The model under review builds one solid part; all positions refer to its coordinate system, in mm. Round coordinates to 2 decimals unless told otherwise and drop trailing zeros. Write each loop counter-clockwise with the first axis right and the second up, starting at its lowest first coordinate (ties: lowest second). Pieces come first, ordered by that corner, then holes. Notation, with made-up numbers: (47.25, 25.25) -> (83.25, 25.25) arc R23 cw to (83.25, 53.25) -> close; hole circle Ø9 at (65.5, -32.5). An arc over 180 degrees is marked (long way). Return JSON: item names as keys, results as strings. Group by question number.
1. Take a section at C-C, the plane z = 3.5. Give the number of separate pieces and of enclosed holes in the cut face, then the cut area to 3 significant figures.
2. Take a section at A-A, the plane x = 42.25. Write out the cut boundary in (y, z), then the cut area to 3 significant figures.
3. For line 1 along X through (y, z) = (-14.5, 0.5) (3 decimals); line 2 along Y through (x, z) = (-2.15, 2.75); line 3 along X through (y, z) = (14, 5), list the stretches that pass through material, from the lowest coordinate up. Write a range as from..to.
4. Take a section at B-B, the plane y = 15. Write out the cut boundary in (x, z), then the cut area to 3 significant figures.
Autodesk Fusion 360 part; units mm, degrees
sketch "Esquisse1" plane through (0, 0, 0) normal (0, 0, 1) x (1, 0, 0)
  line L0 (-35, 50) -> (75, 50)
  line L1 (75, 50) -> (75, -35)
  line L2 (75, -35) -> (-35, -35)
  line L3 (-35, -35) -> (-35, 50)
  circle A0 centre (28.055, -5) radius 2.5
  circle A1 centre (-2.15, 18) radius 1.25
  circle A2 centre (15.555, -5) radius 2.5
  circle A3 centre (-2.15, -3) radius 1.25
  circle A4 centre (15.555, 20) radius 2.5
  circle A5 centre (42.25, 7.5) radius 1.25
  circle A6 centre (28.055, 20) radius 2.5
  line L4 (-11.4, 4.8329) -> (-6.4, 4.8329)
  line L5 (-11.4, 7.8329) -> (-6.4, 7.8329)
  line L6 (15.3682, 31.55) -> (15.3682, 26.55)
  line L7 (18.3682, 31.55) -> (18.3682, 26.55)
  line L8 (46.4, 10) -> (51.4, 10)
  line L9 (46.4, 7) -> (51.4, 7)
  line L10 (15.555, -11.55) -> (15.555, -16.55)
  line L11 (18.555, -11.55) -> (18.555, -16.55)
  line L12 (-11.4, 31.55) -> (15.3682, 31.55)
  line L13 (18.3682, 31.55) -> (51.4, 31.55)
  line L14 (46.4, 26.55) -> (18.3682, 26.55)
  line L15 (15.3682, 26.55) -> (-6.4, 26.55)
  line L16 (51.4, 31.55) -> (51.4, 10)
  line L17 (51.4, 7) -> (51.4, -16.55)
  line L18 (46.4, -11.55) -> (46.4, 7)
  line L19 (46.4, 10) -> (46.4, 26.55)
  line L20 (-6.4, -11.55) -> (15.555, -11.55)
  line L21 (18.555, -11.55) -> (46.4, -11.55)
  line L22 (51.4, -16.55) -> (18.555, -16.55)
  line L23 (15.555, -16.55) -> (-11.4, -16.55)
  line L24 (-11.4, -16.55) -> (-11.4, 4.8329)
  line L25 (-11.4, 7.8329) -> (-11.4, 31.55)
  line L26 (-6.4, 26.55) -> (-6.4, 7.8329)
  line L27 (-6.4, 4.8329) -> (-6.4, -11.55)
  point P0 (20, 10)
  dimension "d1" = 110
  dimension "d2" = 85
  dimension "d3" = 2.5
  dimension "d4" = 2.5
  dimension "d5" = 5
  dimension "d6" = 5
  dimension "d7" = 5
  dimension "d8" = 5
  dimension "d9" = 2.5
  dimension "d10" = 38.1
  dimension "d11" = 52.8
  dimension "d12" = 6.55
  dimension "d13" = 6.55
  dimension "d14" = 8.55
  dimension "d15" = 8.55
  dimension "d16" = 6.55
  dimension "d17" = 6.55
  dimension "d18" = 19.05
  dimension "d19" = 4.15
  dimension "d20" = 18.345
  dimension "d21" = 30.845
  dimension "d22" = 4.25
  dimension "d23" = 4.25
  dimension "d24" = 21.955
  dimension "d25" = 18.345
  dimension "d26" = 23.45
  dimension "d27" = 38.1
  dimension "d28" = 52.8
  dimension "d30" = 28.6
  dimension "d35" = 5
  dimension "d36" = 5
  dimension "d37" = 5
  dimension "d38" = 5
  dimension "d39" = 3
  dimension "d40" = 3
  dimension "d41" = 3
  dimension "d42" = 3
extrude "Extrusion3" add sketch "Esquisse1" along normal blind 6.5 contours L0 L1 L2 L3 | A1 | A3 | A5
sketch "Esquisse3" plane through (0, 0, 6.5) normal (0, 0, 1) x (-1, 0, 0)
  circle A0 centre (-15.555, -20) radius 2.5
  circle A1 centre (-28.055, -20) radius 2.5
  line L0 (11.4, -4.8329) -> (6.4, -4.8329)
  line L1 (6.4, -4.8329) -> (6.4, 11.55)
  line L2 (6.4, 11.55) -> (-15.555, 11.55)
  line L3 (-15.555, 11.55) -> (-15.555, 16.55)
  line L4 (-15.555, 16.55) -> (11.4, 16.55)
  line L5 (11.4, 16.55) -> (11.4, -4.8329)
  line L6 (-18.3682, -26.55) -> (-18.3682, -31.55)
  line L7 (-18.3682, -31.55) -> (-51.4, -31.55)
  line L8 (-51.4, -31.55) -> (-51.4, -10)
  line L9 (-51.4, -10) -> (-46.4, -10)
  line L10 (-46.4, -10) -> (-46.4, -26.55)
  line L11 (-46.4, -26.55) -> (-18.3682, -26.55)
  circle A2 centre (-28.055, 5) radius 2.5
  line L12 (-18.555, 16.55) -> (-18.555, 11.55)
  line L13 (-18.555, 11.55) -> (-46.4, 11.55)
  line L14 (-46.4, 11.55) -> (-46.4, -7)
  line L15 (-46.4, -7) -> (-51.4, -7)
  line L16 (-51.4, -7) -> (-51.4, 16.55)
  line L17 (-51.4, 16.55) -> (-18.555, 16.55)
  line L18 (6.4, -7.8329) -> (11.4, -7.8329)
  line L19 (11.4, -7.8329) -> (11.4, -31.55)
  line L20 (11.4, -31.55) -> (-15.3682, -31.55)
  line L21 (-15.3682, -31.55) -> (-15.3682, -26.55)
  line L22 (-15.3682, -26.55) -> (6.4, -26.55)
  line L23 (6.4, -26.55) -> (6.4, -7.8329)
  circle A3 centre (-15.555, 5) radius 2.5
  line L24 (35, 35) -> (-75, 35)
  line L25 (-75, 35) -> (-75, -50)
  line L26 (-75, -50) -> (35, -50)
  line L27 (35, -50) -> (35, 35)
  line L28 (6.4, 35) -> (6.4, -50) construction
extrude "Extrusion4" cut sketch "Esquisse1" along normal blind 6.5 contours A1 | A3 | A5
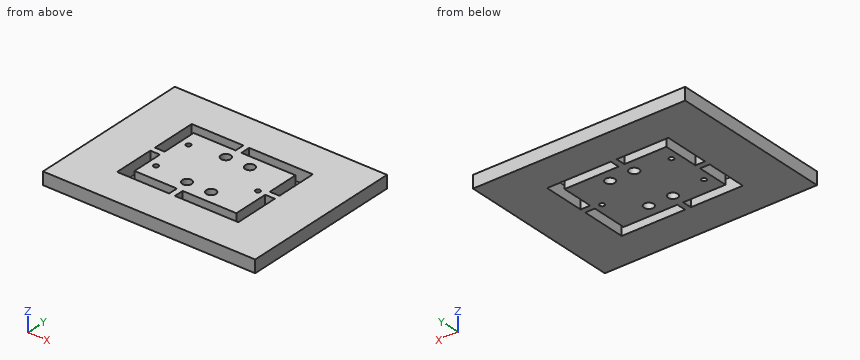
Output:
{
 "1": {"separate pieces": "1", "enclosed holes": "11", "area": "8,310 mm^2"},
 "2": {"outline": "(-35, 0) -> (-16.55, 0) -> (-16.55, 6.5) -> (-35, 6.5) -> close; (-11.55, 0) -> (6.25, 0) -> (6.25, 6.5) -> (-11.55, 6.5) -> close; (8.75, 0) -> (26.55, 0) -> (26.55, 6.5) -> (8.75, 6.5) -> close; (31.55, 0) -> (50, 0) -> (50, 6.5) -> (31.55, 6.5) -> close", "area": "471 mm^2"},
 "3": {"line 1": "x = -35..-11.4, 15.555..18.555, 51.4..75", "line 2": "y = -35..-16.55, -11.55..-4.25, -1.75..16.75, 19.25..26.55, 31.55..50", "line 3": "x = -35..-11.4, -6.4..46.4, 51.4..75"},
 "4": {"outline": "(-35, 0) -> (-11.4, 0) -> (-11.4, 6.5) -> (-35, 6.5) -> close; (-6.4, 0) -> (46.4, 0) -> (46.4, 6.5) -> (-6.4, 6.5) -> close; (51.4, 0) -> (75, 0) -> (75, 6.5) -> (51.4, 6.5) -> close", "area": "650 mm^2"}
}
